Could you check a few things on this model? Use its own coordinates, in mm. Face numbers are marked on the shaded views. Round coordinates to 2 decimals unless told otherwise and drop trailing zeros. Loops run counter-clockwise (first coordinate to the right, second up) from the corner with the lowest first, then second, coordinate; pieces in that order, holes last. Notation, with made-up numbers: (80.5, 73) - (84.5, 73) arc R8 ccw to (84.5, 88) - close; hole circle Ø7 at (-32.75, -24). An arc over 180 degrees is marked (long way). Put each result on its own line as item: value. Start each with the question number.
Autodesk Inventor part; units mm, degrees
ref_plane "YZ Plane" through (0, 0, 0) normal (1, 0, 0) x (0, 1, 0)
ref_plane "XZ Plane" through (0, 0, 0) normal (0, 1, 0) x (-1, 0, 0)
ref_plane "XY Plane" through (0, 0, 0) normal (0, 0, 1) x (1, 0, 0)
sketch "Boceto1" plane through (0, 0, 0) normal (0, 0, 1) x (1, 0, 0)
  line L0 (0, 0) -> (9, 0)
  line L1 (9, 0) -> (9, 5)
  line L2 (9, 5) -> (0, 5)
  line L3 (0, 5) -> (0, 0)
  line L4 (-11.6146, 0) -> (11.6146, 0)
  line L5 (0, 0) -> (0, 2.5)
  line L6 (0, 2.5) -> (2.5247, -1.873)
  dimension "d0" = 9
  dimension "d1" = 5
  dimension "d3" = 2.5
  dimension "d4" = 5
  dimension "d5" = 30
revolve "Revolución1" add sketch "Boceto1" angle 360 about axis through (-11.6146, 0, 0) along (1, 0, 0)
chamfer "Chaflán1" distance 2 angle 30 2 edges at (0, -5, 0) (9, -5, 0) measured on face at (6, 4.9838, -0.4023)
sketch "Boceto2" plane through (9, 0, 0) normal (1, 0, 0) x (0, 0, -1)
  circle A0 centre (0, 0) radius 5
  point P0 (0, 0)
hole "Agujero1" at (9, 0, 0) direction (-1, 0, 0) diameter 5 end through all
properties part number "hudson1-37"
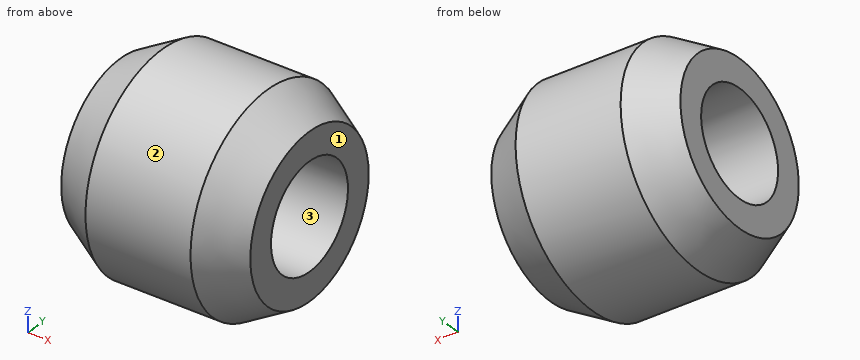
Item 1: I need wall thicknesses on line 1 (Z direction, x = 6.5, y = 0); line 2 (Y direction, x = 5.75, z = -1.75); line 3 (Z direction, x = 2.5, y = -0.75). Which ranges of each line are inside material? Lowest first, please. Write a range as from..to.
Item 2: Thinking about a two-plate mould opening in Y: for the marked faces 1, 2 and 3, which applies, released by +Y, released by -Y, zero draft, split by the parting line, or undercut?
Item 3: Suppose I cut it at C-C, the plane x = 2.5. List the corners of the cut face in (y, z) for me, then the cut area to 3 significant figures.
Item 4: Suppose I cut it at D-D, the plane x = 8.5. List the corners of the cut face in (y, z) for me, then the cut area to 3 significant figures.
Item 5: Will these pins go through, and if not, where does the flat tip stop? P1, Ø1, axis at x = 2.5, z = 2, coming from the +Y side; P2, Ø2, axis at x = 2.5, y = 2.5, coming from the +Z side; P3, Ø4.5, axis at y = 0, z = 0, coming from the -X side; P4, Ø1, axis at x = 3, y = 4, coming from the +Z side.
Item 6: Suppose I cut it at A-A, the plane z = 0. List the corners of the cut face in (x, y) for me.
Numbers:
1. line 1: -5..-2.5, 2.5..5
1. line 2: -4.68..-1.79, 1.79..4.68
1. line 3: -4.94..-2.38, 2.38..4.94
2. face 1: zero draft
2. face 2: split by the parting line
2. face 3: undercut
3. outline: circle Ø10 at (0, 0); hole circle Ø5 at (0, 0)
3. area: 58.9 mm^2
4. outline: circle Ø8.27 at (0, 0); hole circle Ø5 at (0, 0)
4. area: 34.1 mm^2
5. P1: y = 4.77
5. P2: z = 4.77
5. P3: through
5. P4: z = 3.57
6. outline: (0, -3.85) - (2, -5) - (7, -5) - (9, -3.85) - (9, -2.5) - (0, -2.5) - close; (0, 2.5) - (9, 2.5) - (9, 3.85) - (7, 5) - (2, 5) - (0, 3.85) - close
